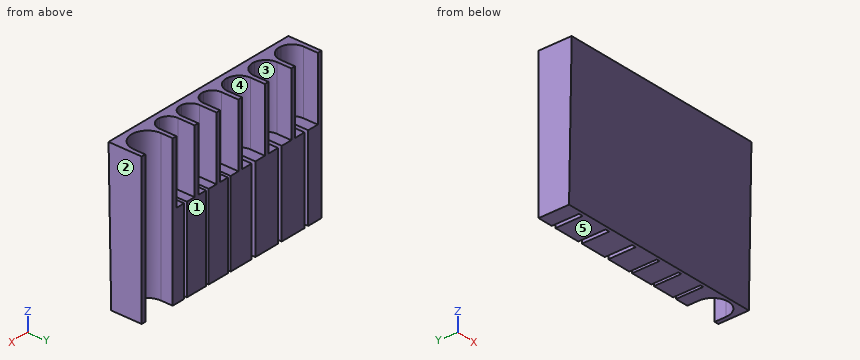
```python
from build123d import *

# Parameters (mm, degrees)
F1_DEPTH = 60
F2_DEPTH = 80
F4_DEPTH = 197
F5_DEPTH = 197


with BuildPart() as f1:
    # F0 (on Top) → F1 (new body)
    with BuildSketch(Plane.XY):
        with BuildLine():
            Line((-176, 30), (-180, 30))
            Line((-180, 30), (-180, 0))
            Line((-180, 0), (0, 0))
            Line((0, 0), (17, 0))
            Line((17, 0), (17, 30))
            Line((17, 30), (13, 30))
            Line((13, 30), (13, 19))
            ThreePointArc((13, 19), (-2, 4), (-17, 19))
            Line((-17, 19), (-17, 30))
            Line((-17, 30), (-21, 30))
            Line((-21, 30), (-21, 14))
            ThreePointArc((-21, 14), (-23.417125, 7.480798), (-29.5, 4.11314))
            ThreePointArc((-29.5, 4.11314), (-31, 4), (-32.5, 4.11314))
            ThreePointArc((-32.5, 4.11314), (-38.582875, 7.480798), (-41, 14))
            Line((-41, 14), (-41, 30))
            Line((-41, 30), (-45, 30))
            Line((-45, 30), (-45, 14))
            ThreePointArc((-45, 14), (-47.417125, 7.480798), (-53.5, 4.11314))
            ThreePointArc((-53.5, 4.11314), (-55, 4), (-56.5, 4.11314))
            ThreePointArc((-56.5, 4.11314), (-62.582875, 7.480798), (-65, 14))
            Line((-65, 14), (-65, 30))
            Line((-65, 30), (-69, 30))
            Line((-69, 30), (-69, 14))
            ThreePointArc((-69, 14), (-71.417125, 7.480798), (-77.5, 4.11314))
            ThreePointArc((-77.5, 4.11314), (-79, 4), (-80.5, 4.11314))
            ThreePointArc((-80.5, 4.11314), (-86.582875, 7.480798), (-89, 14))
            Line((-89, 14), (-89, 30))
            Line((-89, 30), (-93.103136, 30))
            Line((-93.103136, 30), (-93.103136, 18.102423))
            ThreePointArc((-93.103136, 18.102423), (-95.479622, 9.027248), (-103.5, 4.161037))
            ThreePointArc((-103.5, 4.161037), (-105.5, 4), (-107.5, 4.161037))
            ThreePointArc((-107.5, 4.161037), (-115.019716, 8.399074), (-118, 16.5))
            Line((-118, 16.5), (-118, 30))
            Line((-118, 30), (-122, 30))
            Line((-122, 30), (-122, 16.5))
            ThreePointArc((-122, 16.5), (-124.980284, 8.399074), (-132.5, 4.161037))
            ThreePointArc((-132.5, 4.161037), (-134.5, 4), (-136.5, 4.161037))
            ThreePointArc((-136.5, 4.161037), (-144.019716, 8.399074), (-147, 16.5))
            Line((-147, 16.5), (-147, 30))
            Line((-147, 30), (-151, 30))
            Line((-151, 30), (-151, 16.5))
            ThreePointArc((-151, 16.5), (-153.980284, 8.399074), (-161.5, 4.161037))
            ThreePointArc((-161.5, 4.161037), (-163.5, 4), (-165.5, 4.161037))
            ThreePointArc((-165.5, 4.161037), (-173.019716, 8.399074), (-176, 16.5))
            Line((-176, 16.5), (-176, 30))
        make_face()
    extrude(amount=F1_DEPTH)

    # F0 (on Top) → F2 (join)
    with BuildSketch(Plane.XY):
        with BuildLine():
            Line((-176, 30), (-180, 30))
            Line((-180, 30), (-180, 0))
            Line((-180, 0), (0, 0))
            Line((0, 0), (17, 0))
            Line((17, 0), (17, 30))
            Line((17, 30), (13, 30))
            Line((13, 30), (13, 19))
            ThreePointArc((13, 19), (-2, 4), (-17, 19))
            Line((-17, 19), (-17, 30))
            Line((-17, 30), (-21, 30))
            Line((-21, 30), (-21, 14))
            ThreePointArc((-21, 14), (-23.417125, 7.480798), (-29.5, 4.11314))
            ThreePointArc((-29.5, 4.11314), (-31, 4), (-32.5, 4.11314))
            ThreePointArc((-32.5, 4.11314), (-38.582875, 7.480798), (-41, 14))
            Line((-41, 14), (-41, 30))
            Line((-41, 30), (-45, 30))
            Line((-45, 30), (-45, 14))
            ThreePointArc((-45, 14), (-47.417125, 7.480798), (-53.5, 4.11314))
            ThreePointArc((-53.5, 4.11314), (-55, 4), (-56.5, 4.11314))
            ThreePointArc((-56.5, 4.11314), (-62.582875, 7.480798), (-65, 14))
            Line((-65, 14), (-65, 30))
            Line((-65, 30), (-69, 30))
            Line((-69, 30), (-69, 14))
            ThreePointArc((-69, 14), (-71.417125, 7.480798), (-77.5, 4.11314))
            ThreePointArc((-77.5, 4.11314), (-79, 4), (-80.5, 4.11314))
            ThreePointArc((-80.5, 4.11314), (-86.582875, 7.480798), (-89, 14))
            Line((-89, 14), (-89, 30))
            Line((-89, 30), (-93.103136, 30))
            Line((-93.103136, 30), (-93.103136, 18.102423))
            ThreePointArc((-93.103136, 18.102423), (-95.479622, 9.027248), (-103.5, 4.161037))
            ThreePointArc((-103.5, 4.161037), (-105.5, 4), (-107.5, 4.161037))
            ThreePointArc((-107.5, 4.161037), (-115.019716, 8.399074), (-118, 16.5))
            Line((-118, 16.5), (-118, 30))
            Line((-118, 30), (-122, 30))
            Line((-122, 30), (-122, 16.5))
            ThreePointArc((-122, 16.5), (-124.980284, 8.399074), (-132.5, 4.161037))
            ThreePointArc((-132.5, 4.161037), (-134.5, 4), (-136.5, 4.161037))
            ThreePointArc((-136.5, 4.161037), (-144.019716, 8.399074), (-147, 16.5))
            Line((-147, 16.5), (-147, 30))
            Line((-147, 30), (-151, 30))
            Line((-151, 30), (-151, 16.5))
            ThreePointArc((-151, 16.5), (-153.980284, 8.399074), (-161.5, 4.161037))
            ThreePointArc((-161.5, 4.161037), (-163.5, 4), (-165.5, 4.161037))
            ThreePointArc((-165.5, 4.161037), (-173.019716, 8.399074), (-176, 16.5))
            Line((-176, 16.5), (-176, 30))
        make_face()
        with BuildLine():
            Line((-165.5, 30), (-176, 30))
            Line((-176, 30), (-176, 16.5))
            ThreePointArc((-176, 16.5), (-173.019716, 8.399074), (-165.5, 4.161037))
            Line((-165.5, 4.161037), (-165.5, 8.647036))
            Line((-165.5, 8.647036), (-165.5, 30))
        make_face()
        with BuildLine():
            Line((-151, 30), (-161.5, 30))
            Line((-161.5, 30), (-161.5, 11.134194))
            Line((-161.5, 11.134194), (-161.5, 4.161037))
            ThreePointArc((-161.5, 4.161037), (-153.980284, 8.399074), (-151, 16.5))
            Line((-151, 16.5), (-151, 30))
        make_face()
        with BuildLine():
            Line((-136.5, 30), (-147, 30))
            Line((-147, 30), (-147, 16.5))
            ThreePointArc((-147, 16.5), (-144.019716, 8.399074), (-136.5, 4.161037))
            Line((-136.5, 4.161037), (-136.5, 13.265696))
            Line((-136.5, 13.265696), (-136.5, 30))
        make_face()
        with BuildLine():
            Line((-122, 30), (-132.5, 30))
            Line((-132.5, 30), (-132.5, 14.049987))
            Line((-132.5, 14.049987), (-132.5, 4.161037))
            ThreePointArc((-132.5, 4.161037), (-124.980284, 8.399074), (-122, 16.5))
            Line((-122, 16.5), (-122, 30))
        make_face()
        with BuildLine():
            Line((-107.5, 30), (-118, 30))
            Line((-118, 30), (-118, 16.5))
            ThreePointArc((-118, 16.5), (-115.019716, 8.399074), (-107.5, 4.161037))
            Line((-107.5, 4.161037), (-107.5, 11.18967))
            Line((-107.5, 11.18967), (-107.5, 30))
        make_face()
        with BuildLine():
            Line((-93.103136, 30), (-103.5, 30))
            Line((-103.5, 30), (-103.5, 10.63935))
            Line((-103.5, 10.63935), (-103.5, 4.161037))
            ThreePointArc((-103.5, 4.161037), (-95.479622, 9.027248), (-93.103136, 18.102423))
            Line((-93.103136, 18.102423), (-93.103136, 30))
        make_face()
        with BuildLine():
            Line((-80.5, 30), (-89, 30))
            Line((-89, 30), (-89, 14))
            ThreePointArc((-89, 14), (-86.582875, 7.480798), (-80.5, 4.11314))
            Line((-80.5, 4.11314), (-80.5, 18.017488))
            Line((-80.5, 18.017488), (-80.5, 30))
        make_face()
        with BuildLine():
            Line((-69, 30), (-77.5, 30))
            Line((-77.5, 30), (-77.5, 17.524529))
            Line((-77.5, 17.524529), (-77.5, 4.11314))
            ThreePointArc((-77.5, 4.11314), (-71.417125, 7.480798), (-69, 14))
            Line((-69, 14), (-69, 30))
        make_face()
        with BuildLine():
            Line((-56.5, 10.179425), (-56.5, 30))
            Line((-56.5, 30), (-65, 30))
            Line((-65, 30), (-65, 14))
            ThreePointArc((-65, 14), (-62.582875, 7.480798), (-56.5, 4.11314))
            Line((-56.5, 4.11314), (-56.5, 10.179425))
        make_face()
        with BuildLine():
            Line((-45, 14), (-45, 30))
            Line((-45, 30), (-53.5, 30))
            Line((-53.5, 30), (-53.5, 10.014313))
            Line((-53.5, 10.014313), (-53.5, 4.11314))
            ThreePointArc((-53.5, 4.11314), (-47.417125, 7.480798), (-45, 14))
        make_face()
        with BuildLine():
            Line((-32.5, 17.372157), (-32.5, 30))
            Line((-32.5, 30), (-41, 30))
            Line((-41, 30), (-41, 14))
            ThreePointArc((-41, 14), (-38.582875, 7.480798), (-32.5, 4.11314))
            Line((-32.5, 4.11314), (-32.5, 17.372157))
        make_face()
        with BuildLine():
            Line((-21, 14), (-21, 30))
            Line((-21, 30), (-29.5, 30))
            Line((-29.5, 30), (-29.5, 17.21671))
            Line((-29.5, 17.21671), (-29.5, 4.11314))
            ThreePointArc((-29.5, 4.11314), (-23.417125, 7.480798), (-21, 14))
        make_face()
    extrude(amount=-F2_DEPTH)

    # F3 (on face) → F4 (join, through all)
    with BuildSketch(Plane(origin=(-180, 0, 0), x_dir=(0, -1, 0), z_dir=(-1, 0, 0))):
        Polygon((0, -24), (1.5, 60), (0, 60), align=None)
    extrude(amount=-F4_DEPTH)

    # F3 (on face) → F5 (cut, through all)
    with BuildSketch(Plane(origin=(-180, 0, 0), x_dir=(0, -1, 0), z_dir=(-1, 0, 0))):
        Polygon((0, -80), (0, -24), (-1, -80), align=None)
    extrude(amount=-F5_DEPTH, mode=Mode.SUBTRACT)


solid = f1.part
```
Check sheet for the modelled part. Datum: model origin and axes. Units: mm. Face numbers are marked on the shaded views. A direction names the side the tool comes from. Give positions to 0.01 mm unless a question says otherwise; leave off trailing zeros. Write each loop counter-clockwise with the first axis right and the second up, starting at its lowest first coordinate (ties: lowest second). Pieces come first, ordered by that corner, then holes. Notation, with made-up numbers: (81.25, -22) -> (131.25, -22) arc R12 ccw to (131.25, -9) -> close; hole circle Ø9 at (13.25, 85.5). An arc over 180 degrees is marked (long way). Use CSV: the item, a comma, the result in double quotes. Start each with the question number.
Q1. Cross-section at B-B on x = -140.5. Enter the section's corners in (y, z), and give its area (3 significant figures).
Q2. Tool access check on the marked faces 4 and 5. Record the directions out of +Z, -Z, +X, -X, +Y, -Y that give a thin tool (end or side, any length) a straight path to the whole face; none if there is none.
Q3. Cross-section at C-C on y = 7.5. Count the separate pieces of the cut face and the enclosed holes in it, and give its area (3 significant figures).
Q4. Scan lines: line 1 along Z through (x, y) = (-170.5, 7); line 2 along Y through (x, z) = (-59, 0.5); line 3 along Y through (x, z) = (9.5, -45.5). Record each from-to range of solid material in increasing order.
Q5. Depth check by flat-ended pin: P1, Ø2.5, axis at x = -36, y = 20.5, coming from the +Z side. Enter the tip coordinate at first touch or a pass-through.
Q6. Release check for a two-part mould opening along X. For the marked faces 1, 2 and 3 record: +X half, -X half, draft (parallel to the pull), parting line (faces both ways), or undercut.
Working result:
1,outline,"(-1.5, 60) -> (1, -80) -> (30, -80) -> (30, 0) -> (5.53, 0) -> (5.53, 60) -> close"
1,area,"2,770 mm^2"
2,face 4,"+Z, +Y"
2,face 5,"-Z, +X, -X, +Y, -Y"
3,separate pieces,"8"
3,enclosed holes,"0"
3,area,"17,300 mm^2"
4,line 1,"z = -80 to 0"
4,line 2,"y = -0.44 to 4.83"
4,line 3,"y = 0.38 to 9.37"
5,P1,"stops at z = 0"
6,face 1,"draft"
6,face 2,"+X half"
6,face 3,"undercut"
